```python
from build123d import *

# Parameters (mm, degrees)
SKETCH1_R           = 21
SKETCH1_R_2         = 6
SKETCH1_R_3         = 2.5
BOSS_EXTRUDE1_DEPTH = 16
SKETCH2_W           = 19.556392274
SKETCH2_H           = 10
CHAMFER1_SIZE       = 0.5
CHAMFER2_SIZE       = 0.5


with BuildPart() as part:
    # Sketch1 → Boss-Extrude1 (new body)
    with BuildSketch(Plane(origin=(0, 0, 0), x_dir=(1, 0, 0), z_dir=(0, 1, 0))):
        with Locations(Location((0, 0, 0), (0, 0, 270))):
            Circle(SKETCH1_R)
        with Locations(Location((0, 0, 0), (0, 0, 270))):
            Circle(SKETCH1_R_2, mode=Mode.SUBTRACT)
        with Locations(Location((0, 16, 0), (0, 0, 270))):
            Circle(SKETCH1_R_3, mode=Mode.SUBTRACT)
        with Locations(Location((13.856406461, 8, 0), (0, 0, 270))):
            Circle(SKETCH1_R_3, mode=Mode.SUBTRACT)
        with Locations(Location((13.856406461, -8, 0), (0, 0, 270))):
            Circle(SKETCH1_R_3, mode=Mode.SUBTRACT)
        with Locations(Location((0, -16, 0), (0, 0, 270))):
            Circle(SKETCH1_R_3, mode=Mode.SUBTRACT)
        with Locations(Location((-13.856406461, -8, 0), (0, 0, 270))):
            Circle(SKETCH1_R_3, mode=Mode.SUBTRACT)
        with Locations(Location((-13.856406461, 8, 0), (0, 0, 270))):
            Circle(SKETCH1_R_3, mode=Mode.SUBTRACT)
    extrude(amount=BOSS_EXTRUDE1_DEPTH)

    # Sketch2 → Cut-Revolve1 (revolve, cut)
    with BuildSketch(Plane(origin=(0, 0, 0), x_dir=(0, 0, -1), z_dir=(1, 0, 0))):
        with Locations((20.288576043, 8)):
            Rectangle(SKETCH2_W, SKETCH2_H)
    revolve(axis=Axis((0, 0, 0), (0, 1, 0)), mode=Mode.SUBTRACT)

    # Chamfer1
    chamfer1_edges = [part.edges().sort_by_distance(p)[0] for p in [
        (0, 3, -21),
        (0, 13, -21),
    ]]
    chamfer(chamfer1_edges, length=CHAMFER1_SIZE)

    # Chamfer2
    chamfer2_edges = [part.edges().sort_by_distance(p)[0] for p in [
        (0, 0, -21),
        (0, 16, -21),
    ]]
    chamfer(chamfer2_edges, length=CHAMFER2_SIZE)


solid = part.part
```
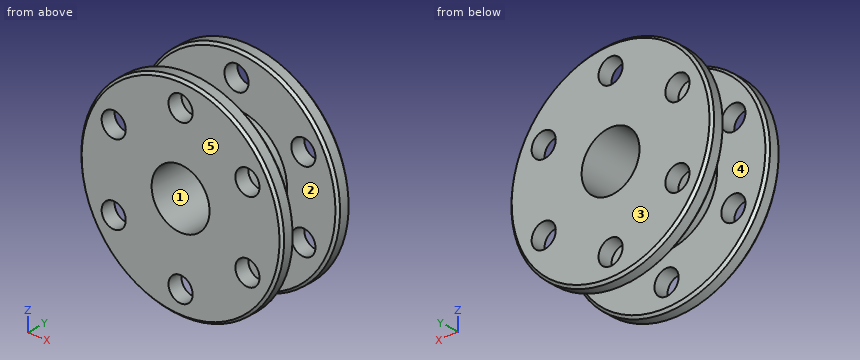
Geometry check sheet. Reference: the model listing, model coordinates, mm. Face numbers are marked on the shaded views. A direction names the side the tool comes from. Round coordinates to 2 decimals unless told otherwise and drop trailing zeros. Loops run counter-clockwise (first coordinate to the right, second up) from the corner with the lowest first, then second, coordinate; pieces in that order, holes last. Notation, with made-up numbers: (53.25, 11) - (98.25, 11) arc R4 cw to (98.25, 15) - close; hole circle Ø7 at (27, 13). An arc over 180 degrees is marked (long way). Write item = value, one per line. Start each with the question number.
1. Section check A-A on z = 0. Enter the section's corners in (x, y).
2. Thickness scan on line 1 (X direction, y = 1.6, z = 8); line 2 (Z direction, x = 15.5, y = 15.25); line 3 (Z direction, x = 1, y = 14.75). Record the ranges inside material, lowest first.
3. Section check B-B on x = 0. Give the number of separate pieces and of enclosed holes in the cut face, then the cut area to 3 significant figures.
4. Mould release check, pull along Y, two halves, no side actions. Record for the marked faces 1, 2 and 3: released by +Y, released by -Y, zero draft, split by the parting line, or undercut.
5. Set-up check for the marked faces 4 and 5: record each of +Z, -Z, +X, -X, +Y, -Y from which the full face is reachable in a straight line by a thin tool's end or side.
6. Depth check by flat-ended pin: pin 1 (1.5 mm diameter, centred on x = -1, y = 7, fed in from +Z); pin 2 (1 mm diameter, centred on x = 15.5, z = 11.5, fed in from -Y); pin 3 (8 mm diameter, centred on x = -6.5, y = 3.5, fed in from +Z); pin 4 (8 mm diameter, centred on y = 10, z = -8.5, fed in from +X). Enter the tip coordinate at first touch or a pass-through.
Working result:
q1.outline = (-21, 0.5) - (-20.5, 0) - (-6, 0) - (-6, 16) - (-20.5, 16) - (-21, 15.5) - (-21, 13.5) - (-20.5, 13) - (-10.51, 13) - (-10.51, 3) - (-20.5, 3) - (-21, 2.5) - close; (6, 0) - (20.5, 0) - (21, 0.5) - (21, 2.5) - (20.5, 3) - (10.51, 3) - (10.51, 13) - (20.5, 13) - (21, 13.5) - (21, 15.5) - (20.5, 16) - (6, 16) - close
q2.line_1 = -19.42 to -16.36, -11.36 to 11.36, 16.36 to 19.42
q2.line_2 = -14.17 to -9.88, -6.12 to 6.12, 9.88 to 14.17
q2.line_3 = -20.98 to -18.29, -13.71 to -5.92, 5.92 to 13.71, 18.29 to 20.98
q3.separate_pieces = 6
q3.enclosed_holes = 0
q3.area = 209 mm^2
q4.face_1 = zero draft
q4.face_2 = undercut
q4.face_3 = released by +Y
q5.face_4 = none
q5.face_5 = +Z, -Z, +X, -X, -Y
q6.pin_1 = 10.51
q6.pin_2 = 0
q6.pin_3 = 20.84
q6.pin_4 = 19.95
